Could you check a few things on this model? Use its own coordinates, in mm. A direction names the side the tool comes from. Give positions to 0.01 mm unless a question says otherwise; leave off trailing zeros. Loops run counter-clockwise (first coordinate to the right, second up) from the corner with the lowest first, then second, coordinate; pieces in that order, holes last. Notation, with made-up numbers: M 78,24.25 L 130,24.25 A30 ccw 130,61.25 Z; hole C 68.5,55.5 d2. An arc over 180 degrees is marked long. Use CSV: the item, a comma, the result in double quotes.
```python
from build123d import *

# Parameters (mm, degrees)
SKETCH1_W                             = 15
SKETCH1_H                             = 52.418
BOSS_EXTRUDE1_DEPTH                   = 45
BOSS_EXTRUDE1_2_DEPTH                 = 45
SKETCH2_W                             = 10.451630362
SKETCH2_H                             = 52.418
SKETCH2_W_2                           = 10
CUT_EXTRUDE1_DEPTH                    = 40
SKETCH3_W                             = 52.418
SKETCH3_H                             = 4.7
BOSS_EXTRUDE3_DEPTH                   = 44
M3_CLEARANCE_HOLE1_D                  = 3.4
M3_CLEARANCE_HOLE1_CSINK_D            = 3.45
M3_CLEARANCE_HOLE1_CSINK_ANGLE        = 90
SKETCH4_R                             = 13.5
CUT_EXTRUDE2_DEPTH                    = 44
TAP_DRILL_FOR_M4X0_7_TAP1_D           = 3.3
TAP_DRILL_FOR_M4X0_7_TAP1_CSINK_D     = 3.35
TAP_DRILL_FOR_M4X0_7_TAP1_CSINK_ANGLE = 90
CHAMFER1_SIZE                         = 10
FILLET1_R                             = 7


with BuildPart() as part:
    # Sketch1 → Boss-Extrude1 (new body)
    with BuildSketch(Plane(origin=(0, 0, 0), x_dir=(1, 0, 0), z_dir=(0, 1, 0))):
        with Locations((7.5, 26.209)):
            Rectangle(SKETCH1_W, SKETCH1_H)
    extrude(amount=BOSS_EXTRUDE1_DEPTH)


with BuildPart() as body_2:
    # Sketch1 → Boss-Extrude1 2 (new body)
    with BuildSketch(Plane(origin=(0, 0, 0), x_dir=(1, 0, 0), z_dir=(0, 1, 0))):
        with Locations((-50.5, 26.209)):
            Rectangle(SKETCH1_W, SKETCH1_H)
    extrude(amount=BOSS_EXTRUDE1_2_DEPTH)


with BuildPart() as cut_extrude1_tool:
    # Sketch2 → Cut-Extrude1 (new body)
    with BuildSketch(Plane(origin=(0, 45, 0), x_dir=(1, 0, 0), z_dir=(0, 1, 0))):
        with Locations((-52.774184819, 26.209)):
            Rectangle(SKETCH2_W, SKETCH2_H)
        with Locations((10, 26.209)):
            Rectangle(SKETCH2_W_2, SKETCH2_H)
    extrude(amount=-CUT_EXTRUDE1_DEPTH)


with BuildPart() as part_1:
    add(part.part)

    # Cut-Extrude1: cut by cut_extrude1_tool
    add(cut_extrude1_tool.part, mode=Mode.SUBTRACT)



with BuildPart() as body_2_1:
    add(body_2.part)

    # Cut-Extrude1: cut by cut_extrude1_tool
    add(cut_extrude1_tool.part, mode=Mode.SUBTRACT)


with BuildPart() as part_2:
    add(part_1.part)

    add(body_2_1.part)  # Boss-Extrude3 merges body 2
    # Sketch3 → Boss-Extrude3 (add)
    with BuildSketch(Plane.ZY):
        with Locations((-26.209, 42.65)):
            Rectangle(SKETCH3_W, SKETCH3_H)
    extrude(amount=BOSS_EXTRUDE3_DEPTH)

    # M3 Clearance Hole1 (through all)
    with Locations(Plane(origin=(0, 45, 0), x_dir=(1, 0, 0), z_dir=(0, 1, 0))):
        with Locations((-36.768184819, 41.703), (-5.780184819, 41.703), (-5.780184819, 10.715), (-36.768184819, 10.715)):
            CounterSinkHole(M3_CLEARANCE_HOLE1_D / 2, M3_CLEARANCE_HOLE1_CSINK_D / 2, counter_sink_angle=M3_CLEARANCE_HOLE1_CSINK_ANGLE)

    # Sketch4 → Cut-Extrude2 (cut)
    with BuildSketch(Plane(origin=(0, 45, 0), x_dir=(1, 0, 0), z_dir=(0, 1, 0))):
        with Locations(Location((-21.274184819, 26.209, 0), (0, 0, 270))):
            Circle(SKETCH4_R)
    extrude(amount=-CUT_EXTRUDE2_DEPTH, mode=Mode.SUBTRACT)

    # Tap Drill for M4x0.7 Tap1 (through all)
    with Locations(Plane(origin=(0, 5, 0), x_dir=(1, 0, 0), z_dir=(0, 1, 0))):
        with Locations((-52.774184819, 26.209), (10, 26.209)):
            CounterSinkHole(TAP_DRILL_FOR_M4X0_7_TAP1_D / 2, TAP_DRILL_FOR_M4X0_7_TAP1_CSINK_D / 2, counter_sink_angle=TAP_DRILL_FOR_M4X0_7_TAP1_CSINK_ANGLE)

    # Chamfer1
    chamfer1_edges = [part_2.edges().sort_by_distance(p)[0] for p in [
        (15, 2.5, -52.418),
        (15, 2.5, 0),
        (-58, 2.5, 0),
        (-58, 2.5, -52.418),
    ]]
    chamfer(chamfer1_edges, length=CHAMFER1_SIZE)

    # Fillet1
    fillet1_edges = [part_2.edges().sort_by_distance(p)[0] for p in [
        (5, 45, -26.209),
        (-47.548369638, 45, -26.209),
    ]]
    fillet(fillet1_edges, radius=FILLET1_R)


solid = part_2.part
```
1. I want a section at B-B, the plane x = 10. List the corners of the cut face in (y, z) for me (3 decimals).
Outcome:
outline,"M 0,-47.418 L 5,-47.418 L 5,-27.884 L 4.975,-27.859 L 0,-27.859 Z; M 0,-24.559 L 4.975,-24.559 L 5,-24.534 L 5,-5 L 0,-5 Z"
2. Which directions (+Z, -Z, +X, -X, +Y, -Y) give clear straight access to the entire face, cutting with the end or side of a thin tool? Please do faces 5 (the face through (8, 5, -27)), 6 (the face through (-53, 2, -5)), 7 (the face through (-47.548, 22, -26)).
Outcome:
face 5,"+Z, -Z, +X, +Y"
face 6,"+Z, -X, +Y, -Y"
face 7,"+Z, -Z, -X, +Y"
3. I want a section at C-C, the plane z = -21. List the corners of the cut face in (x, y) for me, then the cut area to 3 significant figures.
Outcome:
outline,"M -58,0 L -43,0 L -43,40.3 L -33.73,40.3 L -33.73,45 L -40.55,45 A7 ccw -47.55,38 L -47.55,5 L -58,5 Z; M -8.82,40.3 L 0,40.3 L 0,0 L 15,0 L 15,5 L 5,5 L 5,38 A7 ccw -2,45 L -8.82,45 Z"
area,"596 mm2"
4. I want a section at A-A, the plane y = 10. List the corners of the cut face in (x, z) for me, then the cut area to 3 significant figures.
Outcome:
outline,"M -47.55,-52.42 L -43,-52.42 L -43,0 L -47.55,0 Z; M 0,-52.42 L 5,-52.42 L 5,0 L 0,0 Z"
area,"501 mm2"
5. I'm going to push flat-ended pins straight in: pin 1 Ø2 at (y, z) = (35, -43) entering from +X; pin 2 Ø4 at (x, z) = (-36.77, -10.72) entering from +Y; pin 3 Ø3 at (x, z) = (-55, -25.5) entering from +Y; pin 4 Ø2 at (y, z) = (33, -20.5) entering from -X. Where does each tip first touch, or does it pass through?
Outcome:
pin 1,"x = 5"
pin 2,"y = 45"
pin 3,"y = 5"
pin 4,"x = -47.55"
6. Please list where these lines run through material, in increasing order: line 1 (X direction, y = 12, z = -34); line 2 (X direction, y = 3, z = -40); line 3 (Y direction, x = -23, z = -41).
Outcome:
line 1,"-47.55 to -43, 0 to 5"
line 2,"-58 to -43, 0 to 15"
line 3,"40.3 to 45"
7. I want a section at D-D, the plane x = -26. List the corners of the cut face in (y, z) for me, then the cut area to 3 significant figures.
Outcome:
outline,"M 40.3,-52.42 L 45,-52.42 L 45,-38.85 L 40.3,-38.85 Z; M 40.3,-13.56 L 45,-13.56 L 45,0 L 40.3,0 Z"
area,"127 mm2"
8. If we mould it in two halves opening along X, with no side actions, what happens to faces 1 (the face through (-51.126, 2.453, -26.282)), 2 (the face through (-58, 2, -26)), 3 (the face through (-17, 41, -52.418)), 4 (the face through (-36.4, 42.605, -40.043))? For each: +X half, -X half, draft (parallel to the pull), parting line (faces both ways), or undercut.
Outcome:
face 1,"undercut"
face 2,"-X half"
face 3,"draft"
face 4,"undercut"
